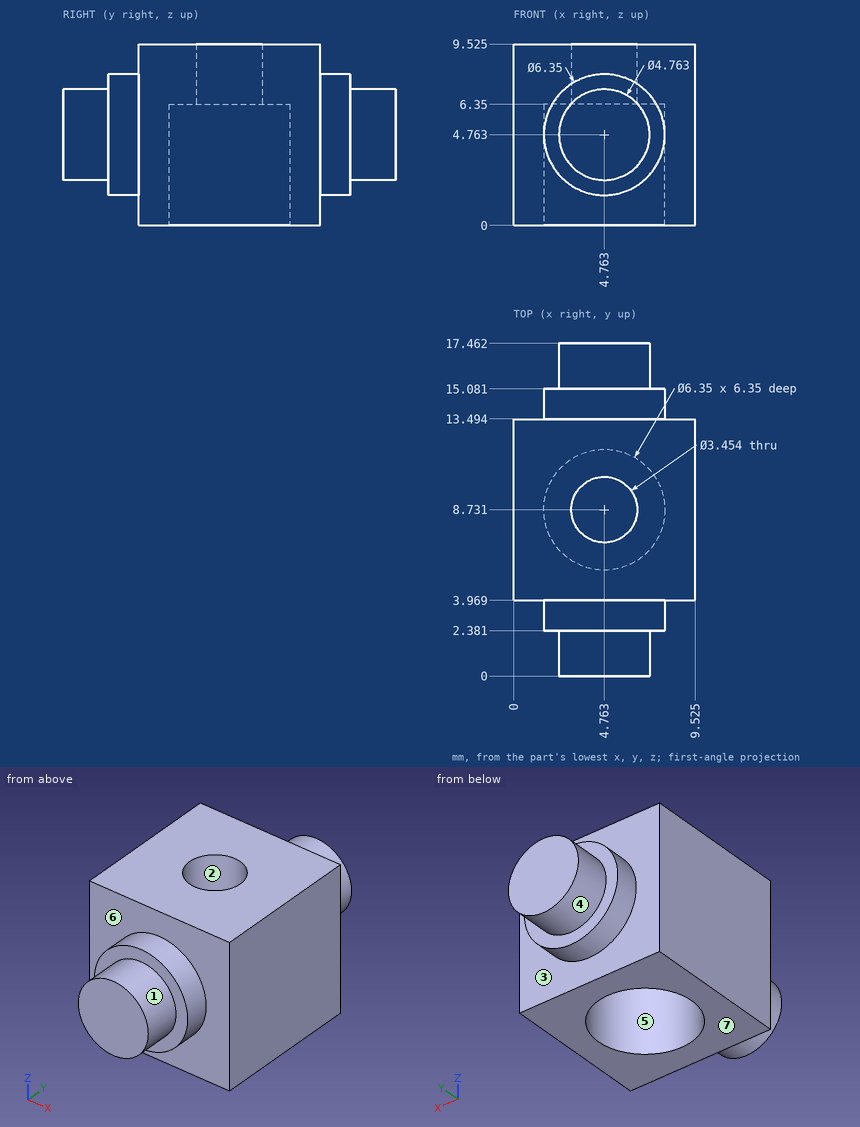
Drawing for the job (mm, zero at the part's lowest x, y, z). A direction names the side the tool comes from. Round coordinates to 2 decimals unless told otherwise and drop trailing zeros. Write item = value, one per line. Start each with the question number.
(1) Pull direction Y, two halves, no side cores. Call the marked faces 1, 2 and 3: released by +Y, released by -Y, zero draft, split by the parting line, or undercut.
(2) Pin check, flat tips, straight feed: P1, Ø5, axis at x = 3.5, z = 5, coming from the -Y side; P2, Ø3, axis at x = 4.5, y = 9, coming from the -Z side. Stop position of each tip, or through.
(3) Probe line 1 (Y direction, x = 0.5, z = 6.5); line 2 (Y direction, x = 7.25, z = 3) (1 decimal); line 3 (Y direction, x = 3, z = 3). List the from-to ranges inside material, lowest first. Write a range as [from, to].
(4) Which spindle directions (+Z, -Z, +X, -X, +Y, -Y) get a long thin tool onto all of the face, cutting with end or side? Do the marked faces 4, 5, 6 and 7. Say none if no direction does.
Model answer:
q1.face_1 = zero draft
q1.face_2 = undercut
q1.face_3 = released by +Y
q2.P1 = 0
q2.P2 = 6.35
q3.line_1 = [3.97, 13.49]
q3.line_2 = [2.4, 6.8], [10.7, 15.1]
q3.line_3 = [2.38, 6.09], [11.37, 15.08]
q4.face_4 = +Y
q4.face_5 = -Z
q4.face_6 = -Y
q4.face_7 = -Z, +X, -X, +Y, -Y
